Verification items for the finished model (mm, model axes). Give positions to 0.01 mm unless a question says otherwise; leave off trailing zeros. Loops run counter-clockwise (first coordinate to the right, second up) from the corner with the lowest first, then second, coordinate; pieces in that order, holes last. Notation, with made-up numbers: M 8.5,27 L 55.5,27 A15 cw 55.5,42 Z; hole C 71,20.25 d6. An arc over 180 degrees is marked long. Answer in a Markdown table with one row per item.
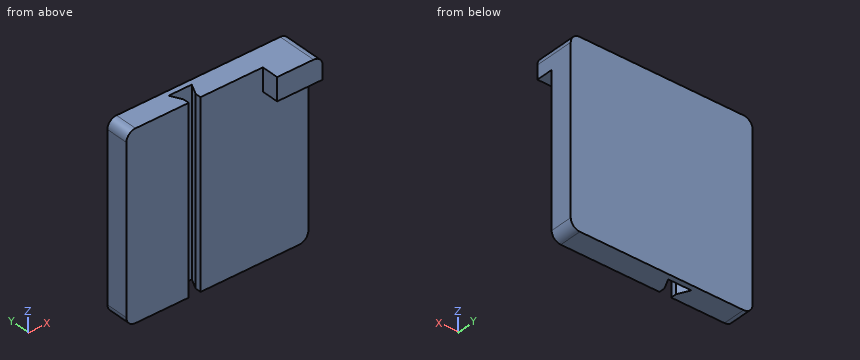
```python
from build123d import *

# Parameters (mm, degrees)
F0_W     = 101.6
F0_H     = 101.6
F1_DEPTH = 12.7
F2_W     = 25.4
F2_H     = 12.7
F3_DEPTH = 9.525
F5_DEPTH = 101.601
F6_R     = 5.08


with BuildPart() as f1:
    # F0 (on Front) → F1 (new body)
    with BuildSketch(Plane.XZ):
        with Locations((50.8, 50.8)):
            Rectangle(F0_W, F0_H)
    extrude(amount=F1_DEPTH)

    # F2 (on face) → F3 (join)
    with BuildSketch(Plane.XZ.offset(12.7)):
        with Locations((88.9, 95.25)):
            Rectangle(F2_W, F2_H)
    extrude(amount=F3_DEPTH)

    # F4 (on face) → F5 (cut, through all)
    with BuildSketch(Plane(origin=(0, 0, 0), x_dir=(1, 0, 0), z_dir=(0, 0, -1))):
        Polygon((41.402, 12.7), (38.1, 12.7), (38.1, 3.048), (44.577, 3.048), (41.402, 9.398), align=None)
        Polygon((38.1, 3.048), (38.1, 12.7), (34.798, 12.7), (34.798, 9.398), (31.623, 3.048), align=None)
    extrude(amount=-F5_DEPTH, mode=Mode.SUBTRACT)

    # F6
    f6_edges = [f1.edges().sort_by_distance(p)[0] for p in [
        (0, -6.35, 101.6),
        (0, -6.35, 0),
        (101.6, -6.35, 0),
        (101.6, -11.1125, 101.6),
    ]]
    fillet(f6_edges, radius=F6_R)


solid = f1.part
```
Item 1: Scan lines: L1, parallel to X at y = -9.75, z = 85; L2, parallel to Y at x = 29, z = 84.5; L3, parallel to X at y = -4.75, z = 69. Record each from-to range of solid material in increasing order. Write a range as [from, to].
Reported:
| item | result |
|---|---|
| L1 | x = [0, 34.8], [41.4, 101.6] |
| L2 | y = [-12.7, 0] |
| L3 | x = [0, 32.47], [43.73, 101.6] |
Item 2: Sectioned sample at B-B (z = 68). Record the cut outline in (x, y), and give its area (3 significant figures).
Reported:
| item | result |
|---|---|
| outline | M 0,-12.7 L 34.8,-12.7 L 34.8,-9.4 L 31.62,-3.05 L 44.58,-3.05 L 41.4,-9.4 L 41.4,-12.7 L 101.6,-12.7 L 101.6,0 L 0,0 Z |
| area | 1,210 mm^2 |
Item 3: Sectioned sample at D-D (x = 83). Record the cut outline in (y, z) (3 decimals), and give its area (3 significant figures).
Reported:
| item | result |
|---|---|
| outline | M -22.225,88.9 L -12.7,88.9 L -12.7,0 L 0,0 L 0,101.6 L -22.225,101.6 Z |
| area | 1,410 mm^2 |
Item 4: Sectioned sample at A-A (y = -11.5). Record the cut outline in (x, z), and give its area (3 significant figures).
Reported:
| item | result |
|---|---|
| outline | M 0,5.08 A5.08 ccw 5.08,0 L 34.8,0 L 34.8,101.6 L 5.08,101.6 A5.08 ccw 0,96.52 Z; M 41.4,0 L 96.52,0 A5.08 ccw 101.6,5.08 L 101.6,96.52 A5.08 ccw 96.52,101.6 L 41.4,101.6 Z |
| area | 9,630 mm^2 |
Item 5: Sectioned sample at C-C (x = 43). Record the cut outline in (y, z), and give its area (3 significant figures).
Reported:
| item | result |
|---|---|
| outline | M -12.7,0 L -6.2,0 L -6.2,101.6 L -12.7,101.6 Z; M -3.05,0 L 0,0 L 0,101.6 L -3.05,101.6 Z |
| area | 970 mm^2 |
Item 6: Go/stop test with flat-tipped pins: pin 1 (3 mm diameter, centred on y = -19.5, z = 93.5, fed in from -X); pin 2 (4 mm diameter, centred on y = -15, z = 79.5, fed in from -X); pin 3 (4 mm diameter, centred on x = 39.5, z = 39.5, fed in from -Y); pin 4 (5 mm diameter, centred on x = 84.5, y = -16.5, fed in from -Z). Record where each tip stops, or that it passes through.
Reported:
| item | result |
|---|---|
| pin 1 | stops at x = 76.2 |
| pin 2 | passes through |
| pin 3 | stops at y = -12.7 |
| pin 4 | stops at z = 88.9 |
